from build123d import *

# Parameters (mm, degrees)
SKETCH1_R           = 4.05
SKETCH1_R_2         = 5
SKETCH1_R_3         = 2.5
BOSS_EXTRUDE1_DEPTH = 10
FILLET1_R           = 11
SKETCH2_R           = 9.05
SKETCH2_R_2         = 4.05
BOSS_EXTRUDE2_DEPTH = 10
FILLET2_R           = 2
SKETCH3_W           = 10
SKETCH3_H           = 60
BOSS_EXTRUDE3_DEPTH = 10
FILLET3_R           = 5
SKETCH4_R           = 1.5
CUT_EXTRUDE1_DEPTH  = 10


with BuildPart() as part:
    # Sketch1 → Boss-Extrude1 (new body)
    with BuildSketch(Plane.XY):
        with BuildLine():
            Line((-80, -12.5), (-51.772571723, -12.5))
            Line((-51.772571723, -12.5), (-40, -17.854919158))
            Line((-40, -17.854919158), (-40, -36.461589484))
            Line((-40, -36.461589484), (40, -36.461589484))
            Line((40, -36.461589484), (40, -12.5))
            Line((40, -12.5), (80, -12.5))
            Line((80, -12.5), (80, 12.5))
            Line((80, 12.5), (25, 12.5))
            Line((25, 12.5), (25, -21.461589484))
            Line((25, -21.461589484), (-25, -21.461589484))
            Line((-25, -21.461589484), (-25, 10.023927765))
            Line((-25, 10.023927765), (-36.337703419, 10.023927765))
            ThreePointArc((-36.337703419, 10.023927765), (-37.531405043, 10.942330613), (-38.821632397, 11.719312422))
            Line((-38.821632397, 11.719312422), (-53.222645277, 19.311460171))
            ThreePointArc((-53.222645277, 19.311460171), (-59.112621671, 18.401196951), (-59.947052977, 12.5))
            Line((-59.947052977, 12.5), (-80, 12.5))
            Line((-80, 12.5), (-80, -12.5))
        make_face()
        with Locations((-67.5, 0)):
            Circle(SKETCH1_R, mode=Mode.SUBTRACT)
        with Locations((67.5, 0)):
            Circle(SKETCH1_R, mode=Mode.SUBTRACT)
        with Locations((-45, 0)):
            Circle(SKETCH1_R_2, mode=Mode.SUBTRACT)
        with Locations((-34.445576532, -14.888473571)):
            Circle(SKETCH1_R_3, mode=Mode.SUBTRACT)
        with Locations((-55.554423468, 14.888473571)):
            Circle(SKETCH1_R_3, mode=Mode.SUBTRACT)
    extrude(amount=BOSS_EXTRUDE1_DEPTH)

    # Fillet1
    fillet1_edges = [part.edges().sort_by_distance(p)[0] for p in [
        (80, 12.5, 5),
        (80, -12.5, 5),
        (40, -12.5, 5),
        (40, -36.461589484, 5),
        (-40, -36.461589484, 5),
        (-40, -17.854919158, 5),
        (-51.772571723, -12.5, 5),
        (-25, 10.023927765, 5),
        (-25, -21.461589484, 5),
        (25, -21.461589484, 5),
        (25, 12.5, 5),
    ]]
    fillet(fillet1_edges, radius=FILLET1_R)

    # Sketch2 → Boss-Extrude2 (add)
    with BuildSketch(Plane.XY.offset(10)):
        with Locations((-67.5, 0)):
            Circle(SKETCH2_R)
        with Locations((-67.5, 0)):
            Circle(SKETCH2_R_2, mode=Mode.SUBTRACT)
        with Locations((67.5, 0)):
            Circle(SKETCH2_R)
        with Locations((67.5, 0)):
            Circle(SKETCH2_R_2, mode=Mode.SUBTRACT)
    extrude(amount=BOSS_EXTRUDE2_DEPTH)

    # Fillet2
    fillet2_edges = [part.edges().sort_by_distance(p)[0] for p in [
        (-76.55, 0, 10),
        (58.45, 0, 10),
    ]]
    fillet(fillet2_edges, radius=FILLET2_R)

    # Sketch3 → Boss-Extrude3 (add)
    with BuildSketch(Plane.ZY.offset(80)):
        with Locations((5, 0)):
            Rectangle(SKETCH3_W, SKETCH3_H)
    extrude(amount=BOSS_EXTRUDE3_DEPTH)

    # Fillet3
    fillet3_edges = [part.edges().sort_by_distance(p)[0] for p in [
        (-80, -12.5, 5),
        (-80, 12.5, 5),
    ]]
    fillet(fillet3_edges, radius=FILLET3_R)

    # Sketch4 → Cut-Extrude1 (cut)
    with BuildSketch(Plane.ZY.offset(90)):
        with Locations((5, 27)):
            Circle(SKETCH4_R)
        with Locations((5, -27)):
            Circle(SKETCH4_R)
    extrude(amount=-CUT_EXTRUDE1_DEPTH, mode=Mode.SUBTRACT)


solid = part.part
Check sheet for the modelled part. Datum: model origin and axes. Units: mm. A direction names the side the tool comes from. Round coordinates to 2 decimals unless told otherwise and drop trailing zeros. Loops run counter-clockwise (first coordinate to the right, second up) from the corner with the lowest first, then second, coordinate; pieces in that order, holes last. Notation, with made-up numbers: (85, 82.25) - (117, 82.25) arc R33 ccw to (117, 117.25) - close; hole circle Ø9 at (77.5, 32.5). An arc over 180 degrees is marked (long way). Answer as CSV lines item,"result". Start each with the question number.
Item 1: Section check C-C (x = -67.5). Record the boundary of the cut face in (y, z).
Item 2: Section check A-A (y = 27). Record the boundary of the cut face in (x, z).
Item 3: Section check B-B (z = 15.75). Record the boundary of the cut face in (x, y), and give its area (3 significant figures).
Item 4: Depth check by flat-ended pin: P1, Ø5, axis at x = 62, z = 6.5, coming from the -Y side; P2, Ø11, axis at y = 21, z = 7, coming from the +X side; P3, Ø8, axis at x = 40, z = 17.5, coming from the +Y side; P4, Ø3.5, axis at y = 27, z = 5, coming from the +X side. Enter the tip coordinate at first touch or a pass-through.
Item 5: Set-up check for faces 1 (the flat face through (-48.046, -14.195, 4.93)), 2 (the flat face through (53, 12.5, 5)), 3 (the cylindrical face through (-78.57, 14, 5.07)): record each of +Z, -Z, +X, -X, +Y, -Y from which the full face is reachable in a straight line by a thin tool's end or side.
Item 6: Release check for a two-part mould opening along Y. For faces 4 (the cylindrical face through (-59.049, 18.464, 4.93)), 5 (the flat face through (60, -12.5, 5)), 6 (the flat face through (-63.6, -1.9, 20)) record: +Y half, -Y half, draft (parallel to the pull), parting line (faces both ways), or undercut.
Item 7: Scan lines: line 1 (X direction, y = 16, z = 6); line 2 (X direction, y = -18, z = 1.75); line 3 (X direction, y = -8, z = 5). Record each from-to range of solid material in increasing order. Write a range as [from, to].
Item 8: Section check D-D (y = -27). Record the boundary of the cut face in (x, z), and give its area (3 significant figures).
Report:
1,outline,"(-12.5, 0) - (-4.05, 0) - (-4.05, 20) - (-9.05, 20) - (-9.05, 12) arc R2 cw to (-11.05, 10) - (-12.5, 10) - close; (4.05, 0) - (12.5, 0) - (12.5, 10) - (11.05, 10) arc R2 cw to (9.05, 12) - (9.05, 20) - (4.05, 20) - close"
2,outline,"(-90, 0) - (-80, 0) - (-80, 3.5) - (-90, 3.5) - close; (-90, 6.5) - (-80, 6.5) - (-80, 10) - (-90, 10) - close"
3,outline,"circle Ø18.1 at (-67.5, 0); circle Ø18.1 at (67.5, 0); hole circle Ø8.1 at (-67.5, 0); hole circle Ø8.1 at (67.5, 0)"
3,area,"412 mm2"
4,P1,"stops at y = -12.5"
4,P2,"stops at x = -45.99"
4,P3,"passes through"
4,P4,"stops at x = -80"
5,face 1,"+Z, -Z, -Y"
5,face 2,"+Z, -Z, +X, +Y"
5,face 3,"+Z, -Z, +Y"
6,face 4,"undercut"
6,face 5,"-Y half"
6,face 6,"draft"
7,line 1,"x = [-90, -79.77], [-60.43, -57.79], [-53.32, -46.94]"
7,line 2,"x = [-90, -80], [-42.46, -22.01], [22.01, 41.47]"
7,line 3,"x = [-90, -25], [25, 77.87]"
8,outline,"(-90, 0) - (-80, 0) - (-80, 3.5) - (-90, 3.5) - close; (-90, 6.5) - (-80, 6.5) - (-80, 10) - (-90, 10) - close; (-39.89, 0) - (39.89, 0) - (39.89, 10) - (-39.89, 10) - close"
8,area,"868 mm2"
